The model under review builds one solid part; all positions refer to its coordinate system, in mm. A direction names the side the tool comes from. Round coordinates to 2 decimals unless told otherwise and drop trailing zeros. Loops run counter-clockwise (first coordinate to the right, second up) from the corner with the lowest first, then second, coordinate; pieces in that order, holes last. Notation, with made-up numbers: (30, -6.75) -> (61, -6.75) arc R22 cw to (61, 3.25) -> close; hole circle Ø1 at (-28, 68.25). An arc over 180 degrees is marked (long way). Write each question's results on one line, items separated by ' | '. Start each with the question number.
Item 1: We need section D-D (z = -22.5). Give the boundary of the cut face in (x, y), and give its area (3 significant figures).
Item 2: For L1, parallel to X at y = -67, z = -39.5; L2, parallel to Z at x = 112.5, y = -31.5; L3, parallel to Y at x = 34, z = -36.5, list the stretches that pass through material, from the lowest coordinate up. Write a range as from..to.
Item 3: Clearance check with flat-ended pins moving along their axes: pin 1 Ø0.5 at (x, z) = (-59, -14.5) entering from +Y; pin 2 Ø3 at (y, z) = (-27.5, 26) entering from -X; pin 3 Ø1.5 at (x, z) = (-30.5, 34) entering from +Y. State where each tip first meets the part, or that it passes through.
Item 4: We need section B-B (x = 5). Give the boundary of the cut face in (y, z), and give its area (3 significant figures).
Item 5: Tool access review of faces 4 (the cylindrical face through (-58.205, -48.936, -54.749)), 5 (the flat face through (53, -99.06, 6)), 6 (the flat face through (-58.586, -26, 6)): name each direction out of +Z, -Z, +X, -X, +Y, -Y from which nothing blocks a thin tool from reaching the whole face with its end or side.
Item 6: We need section A-A (y = -15). Give the boundary of the cut face in (x, z).
Item 7: We need section C-C (z = -0.5). Give the boundary of the cut face in (x, y).
Item 8: Mouldability with a two-part tool opening along X and no side actions: class faces 1 (the flat face through (167.867, -48, 5)), 2 (the flat face through (-57.113, -25, 5)), 3 (the flat face through (54, 0, 65)) as pulls with the +X half, pulls with the -X half, needs draft (parallel to the pull), parting line crosses it, or undercut.
from build123d import *

# Parameters (mm, degrees)
F0_W      = 227.5207936764
F0_H      = 123.2175752521
F1_DEPTH  = 101.6
F2_T      = -2.54
F3_R      = 5.08
F4_R      = 5.08
F5_R      = 5.08
F6_R      = 5.08
F7_R      = 5.08
F8_R      = 5.08
F9_R      = 5.08
F10_R     = 5.08
F11_R     = 5.08
F12_W     = 96.52
F12_H     = 113.0575752521
F12_R     = 21.0345271837
F13_DEPTH = 1.06687
F14_DEPTH = 25.4


with BuildPart() as f1:
    # F0 (on Front) → F1 (new body)
    with BuildSketch(Plane.XZ):
        with Locations((54.1070699692, 5.3321830928)):
            Rectangle(F0_W, F0_H)
    extrude(amount=F1_DEPTH)

    # F2
    f2_openings = [f1.faces().sort_by_distance(p)[0] for p in [
        (54.10707, 0, 5.332183),
    ]]
    offset(amount=F2_T, openings=f2_openings)

    # F3
    f3_edges = [f1.edges().sort_by_distance(p)[0] for p in [
        (54.10707, -99.06, 64.400971),
    ]]
    fillet(f3_edges, radius=F3_R)

    # F4
    f4_edges = [f1.edges().sort_by_distance(p)[0] for p in [
        (-57.113327, -99.06, 2.792183),
    ]]
    fillet(f4_edges, radius=F4_R)

    # F5
    f5_edges = [f1.edges().sort_by_distance(p)[0] for p in [
        (56.64707, -99.06, -53.736605),
    ]]
    fillet(f5_edges, radius=F5_R)

    # F6
    f6_edges = [f1.edges().sort_by_distance(p)[0] for p in [
        (165.327467, -99.06, 5.332183),
    ]]
    fillet(f6_edges, radius=F6_R)

    # F7
    f7_edges = [f1.edges().sort_by_distance(p)[0] for p in [
        (-59.653327, -50.8, 66.940971),
    ]]
    fillet(f7_edges, radius=F7_R)

    # F8
    f8_edges = [f1.edges().sort_by_distance(p)[0] for p in [
        (-59.653327, -50.8, -56.276605),
    ]]
    fillet(f8_edges, radius=F8_R)

    # F9
    f9_edges = [f1.edges().sort_by_distance(p)[0] for p in [
        (167.867467, -50.8, 66.940971),
    ]]
    fillet(f9_edges, radius=F9_R)

    # F10
    f10_edges = [f1.edges().sort_by_distance(p)[0] for p in [
        (162.787467, -50.8, 66.940971),
        (167.867467, -50.8, -56.276605),
    ]]
    fillet(f10_edges, radius=F10_R)

    # F11
    f11_edges = [f1.edges().sort_by_distance(p)[0] for p in [
        (54.10707, -101.6, 66.940971),
    ]]
    fillet(f11_edges, radius=F11_R)

    # F12 (on face) → F13 (cut)
    with BuildSketch(Plane(origin=(-59.653326869, 0, 0), x_dir=(0, -1, 0), z_dir=(-1, 0, 0))):
        with Locations((48.26, 5.3321830928)):
            Rectangle(F12_W, F12_H)
        with Locations((49.5954602957, 6.9027016871)):
            Circle(F12_R, mode=Mode.SUBTRACT)
    extrude(amount=-F13_DEPTH, mode=Mode.SUBTRACT)

    # F14 (cut): a face of the model
    f14_faces = [f1.faces().sort_by_distance(p)[0] for p in [
        (-59.653326869, -49.5954602957, 6.9027016871),
    ]]
    extrude(f14_faces, amount=-F14_DEPTH, mode=Mode.SUBTRACT)


solid = f1.part
Here are the results:
1) outline: (-59.65, -96.52) arc R5.08 ccw to (-54.57, -101.6) -> (162.79, -101.6) arc R5.08 ccw to (167.87, -96.52) -> (167.87, 0) -> (165.33, 0) -> (165.33, -93.98) arc R5.08 cw to (160.25, -99.06) -> (-52.03, -99.06) arc R5.08 cw to (-57.11, -93.98) -> (-57.11, 0) -> (-58.59, 0) -> (-58.59, -96.52) -> close | area: 978 mm2
2) L1: x = -58.59..-57.11, 165.33..167.87 | L2: z = -56.28..-53.74, 64.4..66.94 | L3: y = -101.6..-99.06
3) pin 1: stops at y = -96.52 | pin 2: stops at x = -58.59 | pin 3: stops at y = -99.06
4) outline: (-101.6, -51.2) arc R5.08 ccw to (-96.52, -56.28) -> (0, -56.28) -> (0, -53.74) -> (-93.98, -53.74) arc R5.08 cw to (-99.06, -48.66) -> (-99.06, 59.32) arc R5.08 cw to (-93.98, 64.4) -> (0, 64.4) -> (0, 66.94) -> (-96.52, 66.94) arc R5.08 ccw to (-101.6, 61.86) -> close | area: 816 mm2
5) face 4: -Z, -X, +Y, -Y | face 5: +Y | face 6: -X, +Y
6) outline: (-59.65, -51.2) arc R5.08 ccw to (-54.57, -56.28) -> (162.79, -56.28) arc R5.08 ccw to (167.87, -51.2) -> (167.87, 61.86) arc R5.08 ccw to (162.79, 66.94) -> (-54.57, 66.94) arc R5.08 ccw to (-59.65, 61.86) -> (-58.59, 61.86) -> (-58.59, -51.2) -> close; hole (-57.11, -48.66) arc R5.08 ccw to (-52.03, -53.74) -> (160.25, -53.74) arc R5.08 ccw to (165.33, -48.66) -> (165.33, 59.32) arc R5.08 ccw to (160.25, 64.4) -> (-52.03, 64.4) arc R5.08 ccw to (-57.11, 59.32) -> close
7) outline: (-59.65, -96.52) arc R5.08 ccw to (-54.57, -101.6) -> (162.79, -101.6) arc R5.08 ccw to (167.87, -96.52) -> (167.87, 0) -> (165.33, 0) -> (165.33, -93.98) arc R5.08 cw to (160.25, -99.06) -> (-52.03, -99.06) arc R5.08 cw to (-57.11, -93.98) -> (-57.11, -69.28) -> (-58.59, -69.28) -> (-58.59, -96.52) -> close; (-58.59, -29.91) -> (-57.11, -29.91) -> (-57.11, 0) -> (-58.59, 0) -> close
8) face 1: pulls with the +X half | face 2: undercut | face 3: needs draft
